Input: part model. Units: mm. Frame: model coordinates. Give positions to 0.01 mm unless a question says otherwise; leave off trailing zeros. Loops run counter-clockwise (first coordinate to the right, second up) from the corner with the lowest first, then second, coordinate; pieces in that order, holes last. Notation, with made-up numbers: M 63,-27 L 120,-27 A30 ccw 120,10 Z; hole C -25.75,63.5 d3. An arc over 180 degrees is marked long. One line per item, written item: value. Start each with the question number.
(1) Section B-B on x = -36. Output: boundary loops of the cut face in (y, z).
(2) Ray query, line 1 along X through (y, z) = (-4.5, 0.15); line 2 along X through (y, z) = (-3.25, -0.9); line 3 along Z through (x, y) = (6, 0.75). Return the intervals inside material, ascending. Write a range as from..to.
(3) Pin query (flat end, axial travel): P1, Ø5, axis at x = -11, y = -3, coming from the +Z side. Return the tip coordinate at first contact, or that it passes through.
(4) Section A-A on z = 0. Output: boundary loops of the cut face in (x, y), plus the area to 3 significant figures.
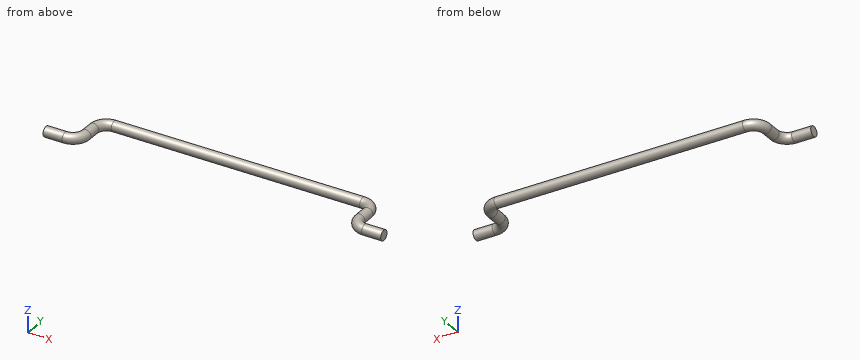
```python
from build123d import *

# Parameters (mm, degrees)
SWEEP2_PROFILE_R = 1.016


with BuildPart() as part:
    # Sweep2: sweep along a path in Sketch12
    with BuildLine(Plane.XY) as sweep2_path:
        Line((15.019045905, -7.62), (11.209045905, -7.62))
        ThreePointArc((11.209045905, -7.62), (9.412994681, -6.876051224), (8.669045905, -5.08))
        Line((8.669045905, -5.08), (8.669045905, -2.54))
        ThreePointArc((8.669045905, -2.54), (7.925097129, -0.743948776), (6.129045905, 0))
        Line((6.129045905, 0), (-38.320954095, 0))
        Line((-38.320954095, 0), (-43.400954095, 0))
        ThreePointArc((-43.400954095, 0), (-45.197005319, -0.743948776), (-45.940954095, -2.54))
        Line((-45.940954095, -2.54), (-45.940954095, -5.08))
        ThreePointArc((-45.940954095, -5.08), (-46.684902871, -6.876051224), (-48.480954095, -7.62))
        Line((-48.480954095, -7.62), (-52.290954095, -7.62))
    # Sweep2 profile (on start of the path) → Sweep2 (sweep)
    with BuildSketch(Plane(origin=(15.019045905, -7.62, 0), x_dir=(0, -1, 0), z_dir=(-1, 0, 0))):
        Circle(SWEEP2_PROFILE_R)
    sweep(path=sweep2_path.line)


solid = part.part
```
Output values:
1. outline: C 0,0 d2.03
2. line 1: x = -46.95..-44.94, 7.66..9.67
2. line 2: x = -46.41..-45.47, 8.2..9.14
2. line 3: z = -0.69..0.69
3. P1: stops at z = 0.88
4. outline: M -52.29,-8.64 L -48.48,-8.64 A3.56 ccw -44.92,-5.08 L -44.92,-2.54 A1.52 cw -43.4,-1.02 L 6.13,-1.02 A1.52 cw 7.65,-2.54 L 7.65,-5.08 A3.56 ccw 11.21,-8.64 L 15.02,-8.64 L 15.02,-6.6 L 11.21,-6.6 A1.52 cw 9.69,-5.08 L 9.69,-2.54 A3.56 ccw 6.13,1.02 L -43.4,1.02 A3.56 ccw -46.96,-2.54 L -46.96,-5.08 A1.52 cw -48.48,-6.6 L -52.29,-6.6 Z
4. area: 159 mm²
